Could you check a few things on this drawing? It's one solid part, dimensions in mm from its lowest x, y, z. A direction names the side the tool comes from. Give positions to 0.01 mm unless a question says otherwise; leave off trailing zeros. Order: outer loops, then holes, each group sorted by start corner. A loop starts at its lowest first (then second) coordinate and runs counter-clockwise, first axis right, second up.
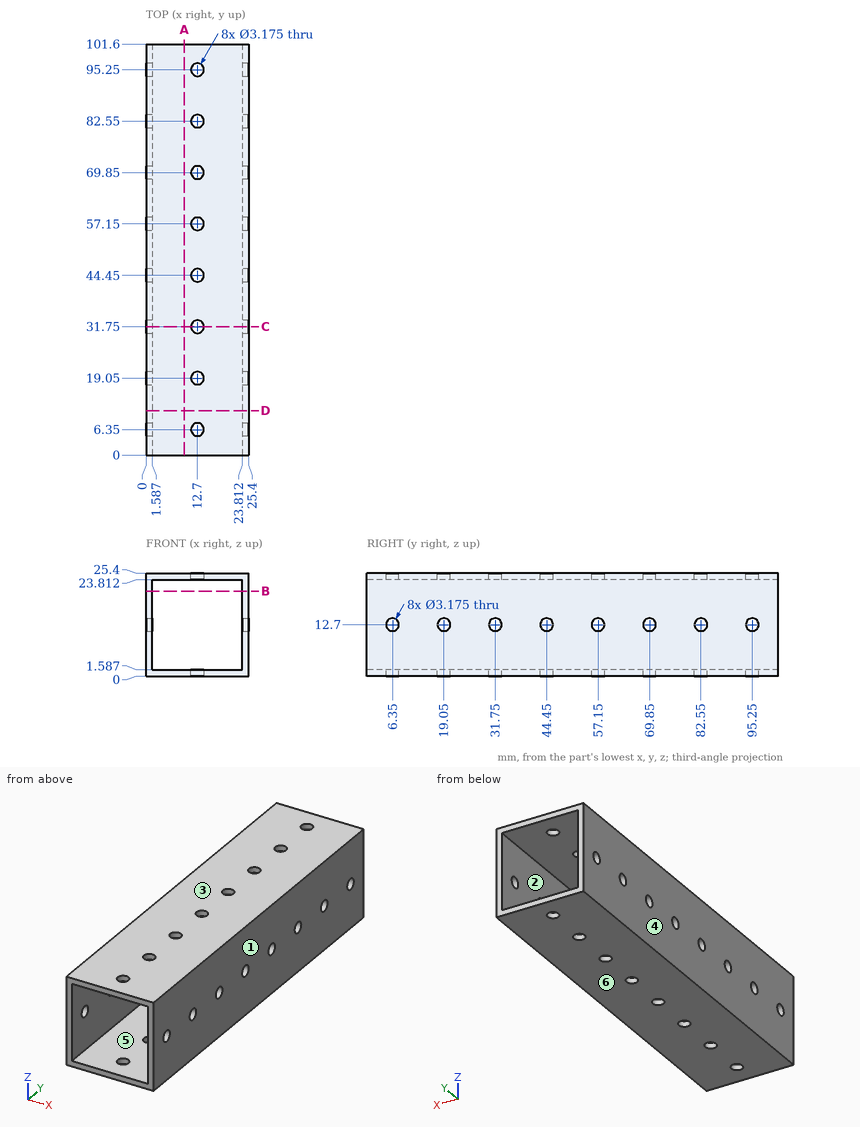
Item 1: For pin 1 (3 mm diameter, centred on x = 12.7, y = 69.85, fed in from +Z), with a flat end and sliding along its axis, tell me the tip position at first contact or that it passes through.
Findings:
pin 1: passes through
Item 2: For the marked faces 1 and 2, which set-ups out of +Z, -Z, +X, -X, +Y, -Y let a thin tool reach every point of the face, with its end or its side?
Findings:
face 1: +Z, -Z, +X, +Y, -Y
face 2: +Y, -Y
Item 3: Imagine slicing it at B-B on z = 21. List the corners of the cut face in (x, y) for me.
Findings:
outline: (0, 0) - (1.59, 0) - (1.59, 101.6) - (0, 101.6) - close; (23.81, 0) - (25.4, 0) - (25.4, 101.6) - (23.81, 101.6) - close
Item 4: Please list where these lines run through material, in increasing order: line 1 along X through (y, z) = (10, 19.75); line 2 along Z through (x, y) = (0.9, 57.15).
Findings:
line 1: x = 0 to 1.59, 23.81 to 25.4
line 2: z = 0 to 11.11, 14.29 to 25.4
Item 5: We'd pull the mould along Z, two halves only. Please class the marked faces 3, 4, 5 and 6: +Z half, -Z half, draft (parallel to the pull), parting line (faces both ways), or undercut.
Findings:
face 3: +Z half
face 4: draft
face 5: undercut
face 6: -Z half
Item 6: Imagine slicing it at C-C on y = 31.75. List the corners of the cut face in (x, z) for me, then the cut area to 3 significant figures.
Findings:
outline: (0, 0) - (11.11, 0) - (11.11, 1.59) - (1.59, 1.59) - (1.59, 11.11) - (0, 11.11) - close; (0, 14.29) - (1.59, 14.29) - (1.59, 23.81) - (11.11, 23.81) - (11.11, 25.4) - (0, 25.4) - close; (14.29, 0) - (25.4, 0) - (25.4, 11.11) - (23.81, 11.11) - (23.81, 1.59) - (14.29, 1.59) - close; (14.29, 23.81) - (23.81, 23.81) - (23.81, 14.29) - (25.4, 14.29) - (25.4, 25.4) - (14.29, 25.4) - close
area: 131 mm2
Item 7: Imagine slicing it at A-A on x = 9.5. List the corners of the cut face in (y, z) for me.
Findings:
outline: (0, 0) - (101.6, 0) - (101.6, 1.59) - (0, 1.59) - close; (0, 23.81) - (101.6, 23.81) - (101.6, 25.4) - (0, 25.4) - close
Item 8: Imagine slicing it at D-D on y = 11. List the corners of the cut face in (x, z) for me.
Findings:
outline: (0, 0) - (25.4, 0) - (25.4, 25.4) - (0, 25.4) - close; hole (1.59, 1.59) - (23.81, 1.59) - (23.81, 23.81) - (1.59, 23.81) - close
